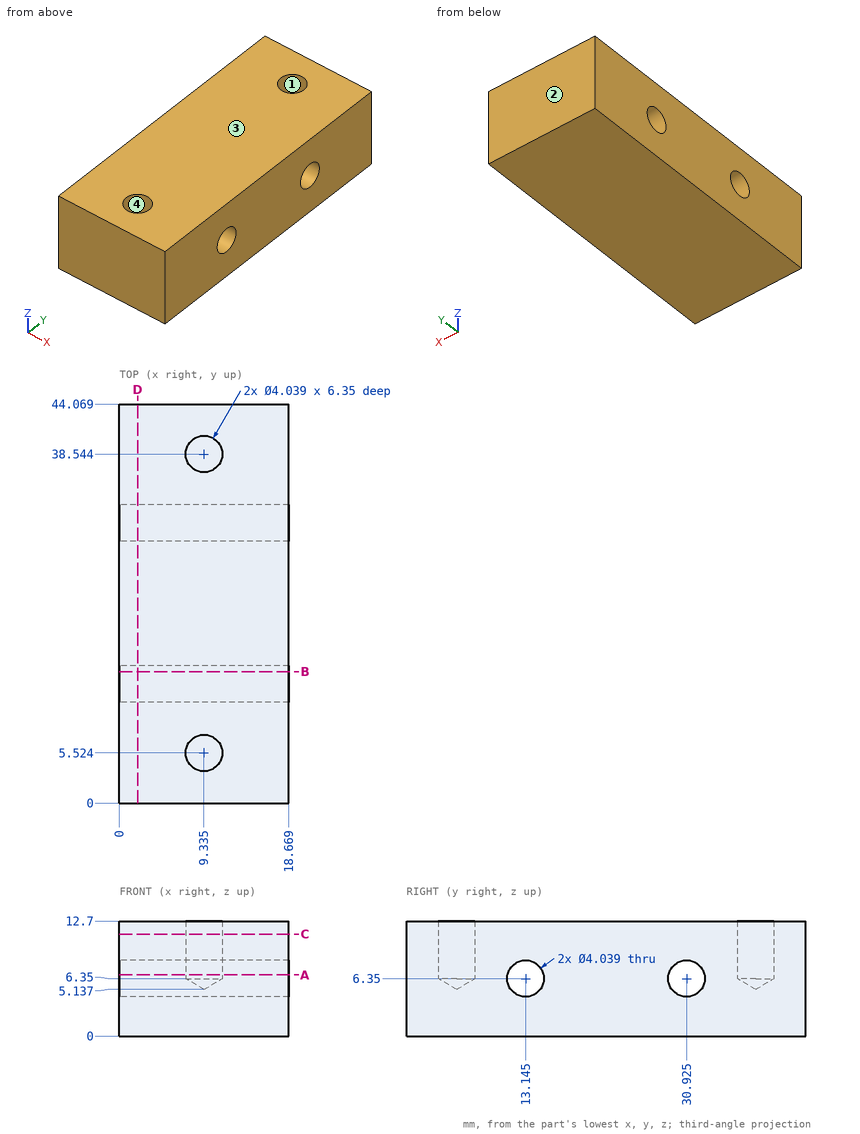
Design review of the part shown in the three views and the two pictorial views. Dimensions are in mm from the part's minimum x, y and z. Round coordinates to 2 decimals unless told otherwise and drop trailing zeros. Write each loop counter-clockwise with the first axis right and the second up, starting at its lowest first coordinate (ties: lowest second). Pieces come first, ordered by that corner, then holes.
1) For line 1 along Y through (x, z) = (4.75, 6.35) (1 decimal); line 2 along Y through (x, z) = (1.5, 5) (1 decimal); line 3 along Y through (x, z) = (9.5, 6.25) (1 decimal), list the stretches that pass through material, from the lowest coordinate up.
Answer below:
line 1: y = 0 to 11.1, 15.2 to 28.9, 32.9 to 44.1
line 2: y = 0 to 11.6, 14.6 to 29.4, 32.4 to 44.1
line 3: y = 0 to 3.7, 7.4 to 11.1, 15.2 to 28.9, 32.9 to 36.7, 40.4 to 44.1
2) Take a section at B-B on y = 14.5. Give the boundary of the cut face in (x, z).
Answer below:
outline: (0, 0) - (18.67, 0) - (18.67, 4.85) - (0, 4.85) - close; (0, 7.85) - (18.67, 7.85) - (18.67, 12.7) - (0, 12.7) - close
3) Mouldability with a two-part tool opening along Y and no side actions: class the marked faces 1, 2, 3 and 4 as +Y half, -Y half, draft (parallel to the pull), parting line (faces both ways), or undercut.
Answer below:
face 1: undercut
face 2: +Y half
face 3: draft
face 4: undercut
4) Insertion check: pin 1 Ø3 at (x, y) = (9.33, 5.52) entering from +Z; pin 2 Ø2.5 at (y, z) = (13.14, 6.35) entering from -X (3 decimals). Each pin has a flat end and moves straight along its axis. Give the tip position at first contact, or say it passes through.
Answer below:
pin 1: stops at z = 6.04
pin 2: passes through
5) Take a section at D-D on x = 2. State how many separate pieces and enclosed holes the cut face has, then the cut area to 3 significant figures.
Answer below:
separate pieces: 1
enclosed holes: 2
area: 534 mm2
6) Take a section at A-A on z = 6.75. Give the boundary of the cut face in (x, y) (1 decimal).
Answer below:
outline: (0, 0) - (18.7, 0) - (18.7, 11.2) - (0, 11.2) - close; (0, 15.1) - (18.7, 15.1) - (18.7, 28.9) - (0, 28.9) - close; (0, 32.9) - (18.7, 32.9) - (18.7, 44.1) - (0, 44.1) - close; hole circle Ø4 at (9.3, 5.5); hole circle Ø4 at (9.3, 38.5)
7) Take a section at C-C on z = 11.25. Give the boundary of the cut face in (x, y) (1 decimal).
Answer below:
outline: (0, 0) - (18.7, 0) - (18.7, 44.1) - (0, 44.1) - close; hole circle Ø4 at (9.3, 5.5); hole circle Ø4 at (9.3, 38.5)
